Part model, mm, in its own coordinate system. Face numbers are marked on the shaded views. A direction names the side the tool comes from. Round coordinates to 2 decimals unless told otherwise and drop trailing zeros. Write each loop counter-clockwise with the first axis right and the second up, starting at its lowest first coordinate (ties: lowest second). Pieces come first, ordered by that corner, then holes. Notation, with made-up numbers: M -30.75,-30 L 8.25,-30 A26 cw 8.25,1 Z; hole C 52,31 d2. An arc over 180 degrees is marked long. Use a Markdown table: item, result. Add a question column.
1) Which spindle directions (+Z, -Z, +X, -X, +Y, -Y) get a long thin tool onto all of the face, cutting with end or side? Do the marked faces 1, 2, 3 and 4. Say none if no direction does.
2) Slice it at C-C on x = -52. Write the cut outline in (y, z), plus the area to 3 significant figures.
3) Slice it at A-A on y = 0. Write the cut outline in (x, z), plus the area to 3 significant figures.
4) Wall check: probe 1 along Y at (x, z) = (-58.5, 4.5); probe 2 along X at (y, z) = (-32, 1.5); probe 3 along X at (y, z) = (56.5, 9.5). Give the ranges that are in metal, low to high.
5) Slice it at B-B on z = 4.25. Write the cut outline in (x, y), plus the area to 3 significant figures.
6) Drop flat-ended pins along their axis: P1, Ø5, axis at x = -36, z = 6.5, coming from the +Y side; P2, Ø3, axis at y = 21.5, z = 5.5, coming from the -X side; P3, Ø3, axis at y = 34.5, z = 2, coming from the -X side. Give the stop position or say it passes through.
7) Slice it at D-D on y = -34.5. Write the cut outline in (x, z).
Autodesk Inventor part; units mm, degrees
ref_plane "YZ Plane" through (0, 0, 0) normal (1, 0, 0) x (0, 1, 0)
ref_plane "XZ Plane" through (0, 0, 0) normal (0, 1, 0) x (-1, 0, 0)
ref_plane "XY Plane" through (0, 0, 0) normal (0, 0, 1) x (1, 0, 0)
sketch "Sketch1" plane through (0, 0, 0) normal (0, 0, 1) x (1, 0, 0)
  line L0 (0, 66.7376) -> (57.7965, 33.3688)
  line L1 (57.7965, 33.3688) -> (57.7965, -33.3688)
  line L2 (57.7965, -33.3688) -> (0, -66.7376)
  line L3 (0, -66.7376) -> (-57.7965, -33.3688)
  line L4 (-57.7965, -33.3688) -> (-57.7965, 33.3688)
  line L5 (-57.7965, 33.3688) -> (0, 66.7376)
  line L6 (-57.7965, 15) -> (-67.7965, 15)
  line L7 (-67.7965, 15) -> (-67.7965, -15)
  line L8 (-67.7965, -15) -> (-57.7965, -15)
  line L9 (-57.7965, -15) -> (-57.7965, 15)
  line L10 (57.7965, 15) -> (67.7965, 15)
  line L11 (67.7965, 15) -> (67.7965, -15)
  line L12 (67.7965, -15) -> (57.7965, -15)
  line L13 (57.7965, -15) -> (57.7965, 15)
  circle A0 centre (-62.7965, 0) radius 3
  circle A1 centre (62.7965, 0) radius 3
  point P0 (0, 0)
  point P1 (0, 0)
  point P2 (-57.7965, 0)
  point P3 (57.7965, 0)
  point P4 (62.7965, 15)
  point P5 (-62.7965, 15)
  dimension "d0" = 10
  dimension "d1" = 30
  dimension "d2" = 30
  dimension "d3" = 10
  dimension "d4" = 133.4752
  dimension "d5" = 6
  dimension "d6" = 6
extrude "Extrusion1" add sketch "Sketch1" along normal blind 10
sketch "Sketch2" plane through (0, 0, 10) normal (0, 0, 1) x (1, 0, 0)
  circle A0 centre (62.7965, 0) radius 3
  circle A1 centre (-62.7965, 0) radius 3
  line L0 (-57.7965, 15) -> (-67.7965, 15)
  line L1 (-67.7965, 15) -> (-67.7965, -15)
  line L2 (-67.7965, -15) -> (-57.7965, -15)
  line L3 (-57.7965, -15) -> (-57.7965, -33.3688)
  line L4 (-57.7965, -33.3688) -> (0, -66.7376)
  line L5 (0, -66.7376) -> (57.7965, -33.3688)
  line L6 (57.7965, -33.3688) -> (57.7965, -15)
  line L7 (57.7965, -15) -> (67.7965, -15)
  line L8 (67.7965, -15) -> (67.7965, 15)
  line L9 (67.7965, 15) -> (57.7965, 15)
  line L10 (57.7965, 15) -> (57.7965, 33.3688)
  line L11 (57.7965, 33.3688) -> (0, 66.7376)
  line L12 (0, 66.7376) -> (-57.7965, 33.3688)
  line L13 (-57.7965, 33.3688) -> (-57.7965, 15)
  line L14 (-56.7965, 32.7915) -> (0, 65.5829)
  line L15 (0, 65.5829) -> (56.7965, 32.7915)
  line L16 (56.7965, 32.7915) -> (56.7965, 14)
  line L17 (56.7965, 14) -> (66.7965, 14)
  line L18 (66.7965, 14) -> (66.7965, -14)
  line L19 (66.7965, -14) -> (56.7965, -14)
  line L20 (56.7965, -14) -> (56.7965, -32.7915)
  line L21 (56.7965, -32.7915) -> (0, -65.5829)
  line L22 (0, -65.5829) -> (-56.7965, -32.7915)
  line L23 (-56.7965, -32.7915) -> (-56.7965, -14)
  line L24 (-56.7965, -14) -> (-66.7965, -14)
  line L25 (-66.7965, -14) -> (-66.7965, 14)
  line L26 (-66.7965, 14) -> (-56.7965, 14)
  line L27 (-56.7965, 14) -> (-56.7965, 32.7915)
  point P0 (0, 0)
  dimension "d9" = 1
extrude "Extrusion2" cut sketch "Sketch2" against normal through all contours L13 L12 L11 L10 L9 L8 L7 L6 L5 L4 L3 L2 L1 L0
properties part number "TARM16" material "ABS Plastic"
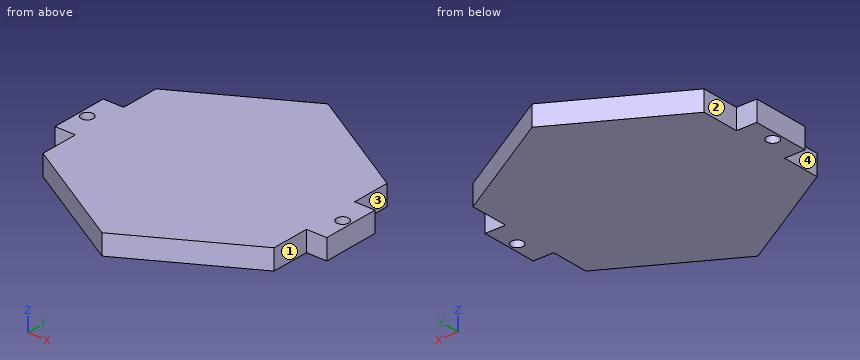
Entries:
| question | item | result |
|---|---|---|
| 1 | face 1 | +Z, -Z, +X, -Y |
| 1 | face 2 | +Z, -Z, -X, +Y |
| 1 | face 3 | +Z, -Z, +X, +Y |
| 1 | face 4 | +Z, -Z, -X, -Y |
| 2 | outline | M -35.56,0 L 35.56,0 L 35.56,10 L -35.56,10 Z |
| 2 | area | 711 mm^2 |
| 3 | outline | M -66.8,0 L -65.8,0 L -65.8,10 L -66.8,10 Z; M -59.8,0 L 59.8,0 L 59.8,10 L -59.8,10 Z; M 65.8,0 L 66.8,0 L 66.8,10 L 65.8,10 Z |
| 3 | area | 1,220 mm^2 |
| 4 | probe 1 | y = -14 to 14 |
| 4 | probe 2 | x = -56.8 to 56.8 |
| 4 | probe 3 | x = -15.73 to 15.73 |
| 5 | outline | M -66.8,-14 L -56.8,-14 L -56.8,-32.79 L 0,-65.58 L 56.8,-32.79 L 56.8,-14 L 66.8,-14 L 66.8,14 L 56.8,14 L 56.8,32.79 L 0,65.58 L -56.8,32.79 L -56.8,14 L -66.8,14 Z; hole C -62.8,0 d6; hole C 62.8,0 d6 |
| 5 | area | 11,700 mm^2 |
| 6 | P1 | stops at y = 46.24 |
| 6 | P2 | stops at x = -56.8 |
| 6 | P3 | stops at x = -56.44 |
| 7 | outline | M -53.84,0 L 53.84,0 L 53.84,10 L -53.84,10 Z |
